Autodesk Inventor part; units mm, degrees
ref_plane "YZ Plane" through (0, 0, 0) normal (1, 0, 0) x (0, 1, 0)
ref_plane "XZ Plane" through (0, 0, 0) normal (0, 1, 0) x (-1, 0, 0)
ref_plane "XY Plane" through (0, 0, 0) normal (0, 0, 1) x (1, 0, 0)
sketch "Sketch1" plane through (0, 0, 0) normal (0, 1, 0) x (-1, 0, 0)
  line L0 (48.5, 48.5) -> (-48.5, 48.5)
  line L1 (-48.5, 48.5) -> (-48.5, -48.5)
  line L2 (-48.5, -48.5) -> (48.5, -48.5)
  line L3 (48.5, -48.5) -> (48.5, 48.5)
  point P0 (0, 0)
  point P1 (48.5, 0)
  point P2 (0, -48.5)
  dimension "d0" = 97
  dimension "d1" = 97
extrude "Extrusion1" add sketch "Sketch1" along normal mid plane 5
sketch "Sketch2" plane through (0, -2.5, 0) normal (0, -1, 0) x (1, 0, 0)
  line L0 (-42.865, 37.465) -> (-42.865, -36.195) construction
  line L1 (42.865, 40.005) -> (42.865, -40.005) construction
  line L2 (-42.865, 6.4948) -> (42.865, 6.4948) construction
  point P0 (0, 0)
  point P1 (42.865, 0)
  point P2 (0, 6.4948)
  dimension "d4" = 73.66
  dimension "d5" = 80.01
  dimension "d6" = 85.73
  dimension "d7" = 3.81
hole "Hole1" at (-42.865, -2.5, 37.465) at (42.865, -2.5, 40.005) at (-42.865, -2.5, -36.195) at (42.865, -2.5, -40.005) direction (0, 1, 0) diameter 3.6 end through all
chamfer "Chamfer1" distance 5 angle 45 4 edges at (48.5, 0, -48.5) (-48.5, 0, -48.5) (48.5, 0, 48.5) (-48.5, 0, 48.5)
sketch "Sketch3" plane through (48.5, -2.5, 43.5) normal (1, 0, 0) x (0, 0, -1)
  point P0 (43.5, 2.5)
  point P1 (71, 2.5)
  point P2 (16, 2.5)
  dimension "d18" = 55
  dimension "d19" = 27.5
hole "Hole2" at (48.5, 0, -27.5) at (48.5, 0, 27.5) direction (-1, 0, 0) diameter 2.1565 depth 4
pattern_circular "Circular Pattern1" count 4 over 360 about axis through (0, -10, 0) along (0, 1, 0) of "Hole2"
sketch "Sketch5" plane through (0, 2.5, 0) normal (0, 1, 0) x (1, 0, 0)
  line L0 (-15, 25) -> (0, 25)
  line L1 (0, 25) -> (0, -25)
  line L2 (0, -25) -> (-15, -25)
  line L3 (-15, -25) -> (-15, 25)
  point P0 (0, 0)
  point P1 (0, 0)
  dimension "d38" = 15
  dimension "d39" = 50
extrude "Extrusion3" cut sketch "Sketch5" against normal through all
sketch "Sketch6" plane through (0, 2.5, 0) normal (0, 1, 0) x (1, 0, 0)
  line L0 (-48.5, 43.5) -> (-48.5, -43.5)
  line L1 (-43.5, 10) -> (-48.5, 10)
  line L2 (-48.5, 10) -> (-48.5, -10)
  line L3 (-48.5, -10) -> (-43.5, -10)
  line L4 (-43.5, -10) -> (-43.5, 10)
  point P0 (0, 0)
  point P1 (-48.5, 0)
  dimension "d42" = 5
  dimension "d43" = 20
extrude "Extrusion4" cut sketch "Sketch6" against normal through all
pattern_circular "Circular Pattern3" count 4 over 360 about axis through (0, -10, 0) along (0, 1, 0) of "Extrusion4"
equation "\"d1\" = d0"
properties part number "stackframesupport" material "Aluminum 6061"
The listing builds one solid part. Answer for the finished solid, in the listing's coordinates (mm). A direction names the side the tool comes from. Give positions to 0.01 mm unless a question says otherwise; leave off trailing zeros. Loops run counter-clockwise (first coordinate to the right, second up) from the corner with the lowest first, then second, coordinate; pieces in that order, holes last. Notation, with made-up numbers: (78.25, 6.5) - (126.25, 6.5) arc R18 ccw to (126.25, 15.5) - close; hole circle Ø6 at (11, 16). An arc over 180 degrees is marked (long way). Write each question's results on one line, items separated by ' | '.
1. For a pull along Y with two mould halves and no side action, classify faces 6 (the face through (-26.5, -1.1, -48.5)), 7 (the face through (-27, 0, -44.5)), 8 (the face through (-26.423, -0.047, -46.472)) as +Y half, -Y half, draft (parallel to the pull), parting line (faces both ways), or undercut.
Resolved:
face 6: draft | face 7: undercut | face 8: undercut
2. Consider probe 1 along X at (y, z) = (-1.1, 21); probe 2 along X at (y, z) = (0, -47.1); probe 3 along X at (y, z) = (1.55, 9). Determine where each line is inside the solid, lowest interval first. Write a range as from..to.
Resolved:
probe 1: x = -48.5..-15, 0..48.5 | probe 2: x = -44.9..-28.58, -26.42..-10, 10..26.42, 28.58..44.9 | probe 3: x = -43.5..-15, 0..43.5
3. Which of the six approach directions +Z, -Z, +X, -X, +Y, -Y give full straight-line access (tool end or side, diameter ignored) to faces 1 (the face through (46, 0, 10)), 2 (the face through (-46, 0, -10)), 3 (the face through (-7, 0, 25)), 4 (the face through (-10, 0, 46)), 5 (the face through (28, 0, -44.5))?
Resolved:
face 1: +X, +Y, -Y | face 2: -X, +Y, -Y | face 3: +Y, -Y | face 4: +Z, +Y, -Y | face 5: -Z
4. Find section B-B, the plane y = 0. Count the separate pieces of the cut face and the enclosed holes in it, then the cut area to 3 significant figures.
Resolved:
separate pieces: 1 | enclosed holes: 5 | area: 8,100 mm^2
5. Find section A-A, the plane z = -8. Write down the section's boundary in (x, y), then the cut area to 3 significant figures.
Resolved:
outline: (-43.5, -2.5) - (-15, -2.5) - (-15, 2.5) - (-43.5, 2.5) - close; (0, -2.5) - (43.5, -2.5) - (43.5, 2.5) - (0, 2.5) - close | area: 360 mm^2
6. Flat-ended cylindrical pins translate along their axes: P1, Ø1.7, axis at x = -27, y = 0.5, coming from the +Z side; P2, Ø1.3, axis at x = -27.5, y = 0, coming from the -Z side; P3, Ø1.5, axis at x = 46.5, y = 1, coming from the +Z side; P4, Ø0.6, axis at y = 0, z = -28, coming from the -X side. Find the tip coordinate at first contact, or state that the pin passes through.
Resolved:
P1: stops at z = 48.5 | P2: stops at z = -44.5 | P3: stops at z = 46.25 | P4: stops at x = -44.5
